```python
from build123d import *

# Parameters (mm, degrees)
SKETCH1_R           = 5
SKETCH1_R_2         = 3
BOSS_EXTRUDE1_DEPTH = 3
SKETCH2_R           = 5.59
SKETCH2_R_2         = 5
BOSS_EXTRUDE2_DEPTH = 0.7
SKETCH3_R           = 4.4
SKETCH3_R_2         = 3.5
CUT_EXTRUDE1_DEPTH  = 0.3
CUT_EXTRUDE2_START  = 0.3
SKETCH4_R           = 4.4
SKETCH4_R_2         = 3.5
CUT_EXTRUDE2_DEPTH  = 0.3


with BuildPart() as part:
    # Sketch1 → Boss-Extrude1 (new body)
    with BuildSketch(Plane(origin=(0, 0, 0), x_dir=(1, 0, 0), z_dir=(0, 1, 0))):
        with Locations(Location((0, 0, 0), (0, 0, 270))):
            Circle(SKETCH1_R)
        with Locations(Location((0, 0, 0), (0, 0, 270))):
            Circle(SKETCH1_R_2, mode=Mode.SUBTRACT)
    extrude(amount=BOSS_EXTRUDE1_DEPTH)

    # Sketch2 → Boss-Extrude2 (add)
    with BuildSketch(Plane(origin=(0, 0, 0), x_dir=(1, 0, 0), z_dir=(0, 1, 0))):
        with Locations(Location((0, 0, 0), (0, 0, 270))):
            Circle(SKETCH2_R)
        with Locations(Location((0, 0, 0), (0, 0, 270))):
            Circle(SKETCH2_R_2, mode=Mode.SUBTRACT)
    extrude(amount=BOSS_EXTRUDE2_DEPTH)

    # Sketch3 → Cut-Extrude1 (cut)
    with BuildSketch(Plane(origin=(0, 3, 0), x_dir=(1, 0, 0), z_dir=(0, 1, 0))):
        with Locations(Location((0, 0, 0), (0, 0, 270))):
            Circle(SKETCH3_R)
        with Locations(Location((0, 0, 0), (0, 0, 270))):
            Circle(SKETCH3_R_2, mode=Mode.SUBTRACT)
    extrude(amount=-CUT_EXTRUDE1_DEPTH, mode=Mode.SUBTRACT)

    # Sketch4 → Cut-Extrude2 (cut)
    with BuildSketch(Plane(origin=(0, 0, 0), x_dir=(1, 0, 0), z_dir=(0, 1, 0)).offset(CUT_EXTRUDE2_START)):
        with Locations(Location((0, 0, 0), (0, 0, 270))):
            Circle(SKETCH4_R)
        with Locations(Location((0, 0, 0), (0, 0, 270))):
            Circle(SKETCH4_R_2, mode=Mode.SUBTRACT)
    extrude(amount=-CUT_EXTRUDE2_DEPTH, mode=Mode.SUBTRACT)


solid = part.part
```
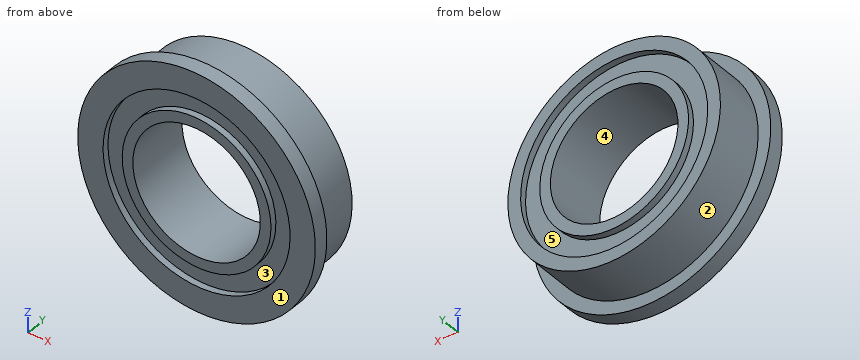
Model file for the job. Use its own axes, mm. Face numbers are marked on the shaded views. A direction names the side the tool comes from. Coordinates: 2 decimals unless noted, no trailing zeros. Loops run counter-clockwise (first coordinate to the right, second up) from the corner with the lowest first, then second, coordinate; pieces in that order, holes last. Notation, with made-up numbers: (40.25, 52) - (73.25, 52) arc R23 ccw to (73.25, 90) - close; hole circle Ø7 at (-18.75, 11). An arc over 180 degrees is marked (long way). Answer as a JSON object with one key per item and string values. Group by question number.
(1) Flat gauge pins, fed straight in: pin 1 (1.5 mm diameter, centred on y = 2, z = 1, fed in from +X); pin 2 (1.5 mm diameter, centred on x = 1, y = 2.5, fed in from -Z); pin 3 (1 mm diameter, centred on y = 1.5, z = 2, fed in from -X). Where does each tip first touch, or does it go through?
(2) Probe line 1 along X through (y, z) = (0.1, 0); line 2 along X through (y, z) = (1.35, 0); line 3 along Z through (x, y) = (0.75, 2.15). List the from-to ranges inside material, lowest first.
(3) Tool access for the marked faces 4 and 5: list every direction of +Z, -Z, +X, -X, +Y, -Y with a clear straight run to the whole face (end or side of a thin tool).
(4) Cut at B-B (z = 0). Give the cut face in (x, y).
(5) Cut at C-C (y = 0.5). Give the cut face in (x, z), then the cut area to 3 significant figures.
(6) Cut at D-D (x = 3.75). Give the cut face in (y, z).
(7) Two-plate mould, pull along Z, no slides. Class the marked faces 1, 2 and 3: released by +Z, released by -Z, zero draft, split by the parting line, or undercut.
(8) Cut at A-A (x = 0). Give the cut face in (y, z).
Geometry says:
{
 "1": {"pin 1": "stops at x = 4.99", "pin 2": "stops at z = -4.99", "pin 3": "stops at x = -4.77"},
 "2": {"line 1": "x = -5.59 to -4.4, -3.5 to -3, 3 to 3.5, 4.4 to 5.59", "line 2": "x = -5 to -3, 3 to 5", "line 3": "z = -4.94 to -2.9, 2.9 to 4.94"},
 "3": {"face 4": "+Y, -Y", "face 5": "+Y"},
 "4": {"outline": "(-5.59, 0) - (-4.4, 0) - (-4.4, 0.3) - (-3.5, 0.3) - (-3.5, 0) - (-3, 0) - (-3, 3) - (-3.5, 3) - (-3.5, 2.7) - (-4.4, 2.7) - (-4.4, 3) - (-5, 3) - (-5, 0.7) - (-5.59, 0.7) - close; (3, 0) - (3.5, 0) - (3.5, 0.3) - (4.4, 0.3) - (4.4, 0) - (5.59, 0) - (5.59, 0.7) - (5, 0.7) - (5, 3) - (4.4, 3) - (4.4, 2.7) - (3.5, 2.7) - (3.5, 3) - (3, 3) - close"},
 "5": {"outline": "circle Ø11.18 at (0, 0); hole circle Ø6 at (0, 0)", "area": "69.9 mm^2"},
 "6": {"outline": "(0, -4.15) - (0.7, -4.15) - (0.7, -3.31) - (3, -3.31) - (3, -2.3) - (2.7, -2.3) - (2.7, 2.3) - (3, 2.3) - (3, 3.31) - (0.7, 3.31) - (0.7, 4.15) - (0, 4.15) - (0, 2.3) - (0.3, 2.3) - (0.3, -2.3) - (0, -2.3) - close"},
 "7": {"face 1": "zero draft", "face 2": "split by the parting line", "face 3": "undercut"},
 "8": {"outline": "(0, -5.59) - (0.7, -5.59) - (0.7, -5) - (3, -5) - (3, -4.4) - (2.7, -4.4) - (2.7, -3.5) - (3, -3.5) - (3, -3) - (0, -3) - (0, -3.5) - (0.3, -3.5) - (0.3, -4.4) - (0, -4.4) - close; (0, 3) - (3, 3) - (3, 3.5) - (2.7, 3.5) - (2.7, 4.4) - (3, 4.4) - (3, 5) - (0.7, 5) - (0.7, 5.59) - (0, 5.59) - (0, 4.4) - (0.3, 4.4) - (0.3, 3.5) - (0, 3.5) - close"}
}
